Input: part model. Units: mm. Frame: model coordinates. Face numbers are marked on the shaded views. A direction names the side the tool comes from. Coordinates: 2 decimals unless noted, no trailing zeros. Order: outer loops, then holes, each group sorted by start corner. A loop starts at its lowest first (then second) coordinate and runs counter-clockwise, first axis right, second up. Notation, with made-up numbers: (-16.75, 71.25) -> (0.25, 71.25) arc R14 ccw to (0.25, 81.25) -> close; hole circle Ø2 at (85.25, 79.25). An arc over 180 degrees is marked (long way). One line per question, with ' | ' between items.
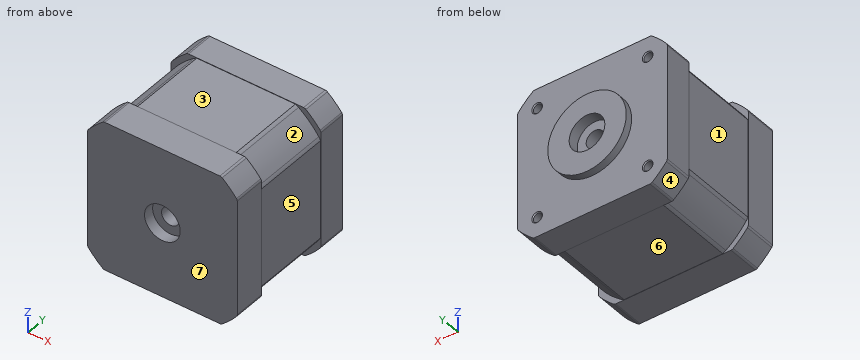
```python
from build123d import *

# Parameters (mm, degrees)
SKETCH2_W          = 55
SKETCH2_H          = 55
SKETCH2_W_2        = 42
SKETCH2_H_2        = 42
CUT_EXTRUDE1_DEPTH = 55.356140408
SKETCH3_W          = 0.1
SKETCH3_H          = 27.678330874
SKETCH3_W_2        = 27.678330874
SKETCH3_H_2        = 0.1
CUT_EXTRUDE2_DEPTH = 22.1
FILLET9_R          = 5
FILLET10_R         = 1
SKETCH4_R          = 1.25
CUT_EXTRUDE3_DEPTH = 6
CHAMFER1_SIZE      = 0.25


with BuildPart() as part:
    # Sketch1 → Revolve1 (revolve)
    with BuildSketch(Plane.XY, mode=Mode.PRIVATE) as revolve1_sk:
        Polygon((5, 0), (11, 0), (11, -2), (26.7, -2), (26.7, -10), (25.15, -10), (25.15, -32.1), (26.7, -32.1), (26.7, -41.1), (5, -41.1), (5, -38.1), (2.5, -38.1), (2.5, -32.1), (11, -32.1), (11, -10), (2.5, -10), (2.5, -3), (5, -3), align=None)
    revolve(revolve1_sk.sketch.rotate(Axis((0, 0, 0), (0, -1, 0)), 180), axis=Axis((0, 0, 0), (0, -1, 0)))

    # Sketch2 → Cut-Extrude1 (cut, through all)
    with BuildSketch(Plane(origin=(0, -2, 0), x_dir=(1, 0, 0), z_dir=(0, 1, 0))):
        Rectangle(SKETCH2_W, SKETCH2_H)
        Rectangle(SKETCH2_W_2, SKETCH2_H_2, mode=Mode.SUBTRACT)
    extrude(amount=-CUT_EXTRUDE1_DEPTH, mode=Mode.SUBTRACT)

    # Sketch3 → Cut-Extrude2 (cut)
    with BuildSketch(Plane.XZ.offset(10)):
        with Locations((-20.95, 0)):
            Rectangle(SKETCH3_W, SKETCH3_H)
        with Locations((0, -20.95)):
            Rectangle(SKETCH3_W_2, SKETCH3_H_2)
        with Locations((20.95, 0)):
            Rectangle(SKETCH3_W, SKETCH3_H)
        with Locations((0, 20.95)):
            Rectangle(SKETCH3_W_2, SKETCH3_H_2)
    extrude(amount=CUT_EXTRUDE2_DEPTH, mode=Mode.SUBTRACT)

    # Fillet9
    # the kernel refuses this fillet: 5 mm, written as the material it takes off along each edge
    with BuildSketch(Plane(origin=(13.839165437, -10, -21), x_dir=(0.8230603738236033, 0, 0.5679538898901478), z_dir=(0, -1, 0)), Plane(origin=(21, -10, 13.839165437), x_dir=(-0.5679538898901461, 0, 0.8230603738236048), z_dir=(0, -1, 0)), Plane(origin=(-13.839165437, -10, 21), x_dir=(-0.8230603738236049, 0, -0.5679538898901455), z_dir=(0, -1, 0)), Plane(origin=(-21, -10, -13.839165437), x_dir=(0.567953889890148, 0, -0.8230603738236033), z_dir=(0, -1, 0))) as fillet9_piece_1:
        with BuildLine():
            CenterArc((0.966453452, 4.998861967), FILLET9_R, 259.51770896, 11.704761359)
            Line((0.056795389, 0.082306037), (0, 0))
            ThreePointArc((0, 0), (0.536563009, -0.005724307), (1.073126019, 0))
        make_face()
    extrude(amount=22.1, mode=Mode.SUBTRACT)
    with BuildSketch(Plane(origin=(21, -10, -13.839165437), x_dir=(-0.5679538898901492, 0, -0.8230603738236025), z_dir=(0, -1, 0)), Plane(origin=(13.839165437, -10, 21), x_dir=(0.8230603738236021, 0, -0.5679538898901498), z_dir=(0, -1, 0)), Plane(origin=(-21, -10, 13.839165437), x_dir=(0.5679538898901505, 0, 0.8230603738236016), z_dir=(0, -1, 0)), Plane(origin=(-13.839165437, -10, -21), x_dir=(-0.8230603738236021, 0, 0.5679538898901498), z_dir=(0, -1, 0))) as fillet9_piece_2:
        with BuildLine():
            CenterArc((0.966453452, -4.998861967), FILLET9_R, 88.777529681, 11.704761359)
            Line((0.056795389, -0.082306037), (0, 0))
            ThreePointArc((0, 0), (0.536563009, 0.005724307), (1.073126019, 0))
        make_face()
    extrude(amount=22.1, mode=Mode.SUBTRACT)

    # Fillet10
    fillet10_edges = [part.edges().sort_by_distance(p)[0] for p in [
        (21, -36.6, -16.4890873),
        (21, -6, -16.4890873),
        (16.4890873, -36.6, 21),
        (16.4890873, -6, 21),
        (-21, -36.6, 16.4890873),
        (-21, -6, 16.4890873),
        (-16.4890873, -36.6, -21),
        (-16.4890873, -6, -21),
        (21, -36.6, 16.4890873),
        (21, -6, 16.4890873),
        (-16.4890873, -36.6, 21),
        (-16.4890873, -6, 21),
        (-21, -36.6, -16.4890873),
        (-21, -6, -16.4890873),
        (16.4890873, -36.6, -21),
        (16.4890873, -6, -21),
    ]]
    fillet(fillet10_edges, radius=FILLET10_R)

    # Sketch4 → Cut-Extrude3 (cut)
    with BuildSketch(Plane(origin=(0, -2, 0), x_dir=(1, 0, 0), z_dir=(0, 1, 0))):
        with Locations(Location((-15.5, 15.5, 0), (0, 0, 180))):
            Circle(SKETCH4_R)
        with Locations(Location((15.5, 15.5, 0), (0, 0, 180))):
            Circle(SKETCH4_R)
        with Locations(Location((15.5, -15.5, 0), (0, 0, 180))):
            Circle(SKETCH4_R)
        with Locations(Location((-15.5, -15.5, 0), (0, 0, 180))):
            Circle(SKETCH4_R)
    extrude(amount=-CUT_EXTRUDE3_DEPTH, mode=Mode.SUBTRACT)

    # Chamfer1
    chamfer1_edges = [part.edges().sort_by_distance(p)[0] for p in [
        (-14.25, -2, -15.5),
        (16.75, -2, -15.5),
        (16.75, -2, 15.5),
        (-14.25, -2, 15.5),
    ]]
    chamfer(chamfer1_edges, length=CHAMFER1_SIZE)


solid = part.part
```
1. Cut plane D-D, the plane z = 15.5. Return loops of the section in (x, y).
Recorded:
outline: (-21, -41.1) -> (21, -41.1) -> (21, -32.1) -> (19.81, -32.1) -> (19.81, -10) -> (21, -10) -> (21, -2) -> (17, -2) -> (16.75, -2.25) -> (16.75, -8) -> (14.25, -8) -> (14.25, -2.25) -> (14, -2) -> (-14, -2) -> (-14.25, -2.25) -> (-14.25, -8) -> (-16.75, -8) -> (-16.75, -2.25) -> (-17, -2) -> (-21, -2) -> (-21, -10) -> (-19.81, -10) -> (-19.81, -32.1) -> (-21, -32.1) -> close
2. Ray query, line 1 (Z direction, x = 15.5, y = -5.3); line 2 (Y direction, x = -5.5, z = 5); line 3 (Y direction, x = 12, z = 13). Return the intervals inside material, ascending. Write a range as [from, to].
Recorded:
line 1: z = [-21, -16.75], [-14.25, 14.25], [16.75, 21] | line 2: y = [-41.1, -32.1], [-10, 0] | line 3: y = [-41.1, -2]
3. Cut plane A-A, the plane y = -18.5. Return loops of the section in (x, z).
Recorded:
outline: (-20.9, -13.84) arc R5 ccw to (-20.39, -14.72) arc R25.15 ccw to (-14.72, -20.39) arc R5 ccw to (-13.84, -20.9) -> (13.84, -20.9) arc R5 ccw to (14.72, -20.39) arc R25.15 ccw to (20.39, -14.72) arc R5 ccw to (20.9, -13.84) -> (20.9, 13.84) arc R5 ccw to (20.39, 14.72) arc R25.15 ccw to (14.72, 20.39) arc R5 ccw to (13.84, 20.9) -> (-13.84, 20.9) arc R5 ccw to (-14.72, 20.39) arc R25.15 ccw to (-20.39, 14.72) arc R5 ccw to (-20.9, 13.84) -> close; hole circle Ø22 at (0, 0)
4. Cut plane C-C, the plane z = 6.5. Return loops of the section in (x, y).
Recorded:
outline: (-21, -41.1) -> (21, -41.1) -> (21, -32.1) -> (20.9, -32.1) -> (20.9, -10) -> (21, -10) -> (21, -2) -> (8.87, -2) -> (8.87, 0) -> (-8.87, 0) -> (-8.87, -2) -> (-21, -2) -> (-21, -10) -> (-20.9, -10) -> (-20.9, -32.1) -> (-21, -32.1) -> close; hole (-8.87, -32.1) -> (8.87, -32.1) -> (8.87, -10) -> (-8.87, -10) -> close
5. Cut plane B-B, the plane x = -12. Return loops of the section in (y, z).
Recorded:
outline: (-41.1, -21) -> (-32.1, -21) -> (-32.1, -20.9) -> (-10, -20.9) -> (-10, -21) -> (-2, -21) -> (-2, 21) -> (-10, 21) -> (-10, 20.9) -> (-32.1, 20.9) -> (-32.1, 21) -> (-41.1, 21) -> close
6. Mould query, pull axis Y, two halves, no side actions, for the marked faces 4, 5, 6 and 7. Classes: released by +Y, released by -Y, zero draft, split by the parting line, or undercut.
Recorded:
face 4: zero draft | face 5: undercut | face 6: undercut | face 7: released by -Y
7. Access query for the marked faces 1, 2 and 3. Directions: +Z, -Z, +X, -X, +Y, -Y. A direction counts if a zero-diameter tool reaches every point of the face in a straight line with its end or side. Return the directions, or none.
Recorded:
face 1: +Z, -Z, -X | face 2: +Z, +X | face 3: +Z, +X, -X
8. Pin query (flat end, axial travel): pin 1 Ø1.5 at (x, y) = (-12, -27) entering from -Z; pin 2 Ø0.8 at (x, z) = (15, -15.5) entering from +Y; pin 3 Ø8 at (x, z) = (0, 0) entering from -Y. Return the tip coordinate at first contact, or that it passes through.
Recorded:
pin 1: stops at z = -20.9 | pin 2: stops at y = -8 | pin 3: stops at y = -38.1
